from build123d import *

# Parameters (mm, degrees)
SKETCH_1_W          = 30
SKETCH_1_H          = 30
EXTRUDE_1_DEPTH     = 10
SKETCH_4_R          = 1.55
CUT_EXTRUDE_1_DEPTH = 30
SKETCH_5_R          = 3.5
SKETCH_5_R_2        = 1.55
CUT_EXTRUDE_2_DEPTH = 3
SKETCH_6_W          = 30
SKETCH_6_H          = 10
EXTRUDE_2_DEPTH     = 16


with BuildPart() as part:
    # 草图1 → 凸台-拉伸1 (new body)
    with BuildSketch(Plane(origin=(0, 0, 0), x_dir=(1, 0, 0), z_dir=(0, 1, 0))):
        Rectangle(SKETCH_1_W, SKETCH_1_H)
    extrude(amount=EXTRUDE_1_DEPTH)

    # 草图4 → 切除-拉伸1 (cut)
    with BuildSketch(Plane.XZ):
        with Locations(Location((5, 1, 0), (0, 0, 270))):
            Circle(SKETCH_4_R)
        with Locations(Location((5, -9, 0), (0, 0, 270))):
            Circle(SKETCH_4_R)
        with Locations(Location((-5, 1, 0), (0, 0, 270))):
            Circle(SKETCH_4_R)
        with Locations(Location((-5, -9, 0), (0, 0, 270))):
            Circle(SKETCH_4_R)
    extrude(amount=-CUT_EXTRUDE_1_DEPTH, mode=Mode.SUBTRACT)

    # 草图5 → 切除-拉伸2 (cut)
    # profile 1 of 4: a face of its own
    with BuildSketch(Plane.XZ):
        with Locations(Location((5, 1, 0), (0, 0, 270))):
            Circle(SKETCH_5_R)
        with Locations(Location((5, 1, 0), (0, 0, 270))):
            Circle(SKETCH_5_R_2, mode=Mode.SUBTRACT)
    # profile 2 of 4: a face of its own
    with BuildSketch(Plane.XZ):
        with Locations(Location((5, -9, 0), (0, 0, 270))):
            Circle(SKETCH_5_R)
        with Locations(Location((5, -9, 0), (0, 0, 270))):
            Circle(SKETCH_5_R_2, mode=Mode.SUBTRACT)
    # profile 3 of 4: a face of its own
    with BuildSketch(Plane.XZ):
        with Locations(Location((-5, -9, 0), (0, 0, 270))):
            Circle(SKETCH_5_R)
        with Locations(Location((-5, -9, 0), (0, 0, 270))):
            Circle(SKETCH_5_R_2, mode=Mode.SUBTRACT)
    # profile 4 of 4: a face of its own
    with BuildSketch(Plane.XZ):
        with Locations(Location((-5, 1, 0), (0, 0, 270))):
            Circle(SKETCH_5_R)
    extrude(amount=-CUT_EXTRUDE_2_DEPTH, mode=Mode.SUBTRACT)

    # 草图6 → 凸台-拉伸2 (add)
    with BuildSketch(Plane.XY.offset(15)):
        with Locations((0, 5)):
            Rectangle(SKETCH_6_W, SKETCH_6_H)
    extrude(amount=EXTRUDE_2_DEPTH)


solid = part.part
The listing builds one solid part. Answer for the finished solid, in the listing's coordinates (mm). A direction names the side the tool comes from. Coordinates: 2 decimals unless noted, no trailing zeros. Order: outer loops, then holes, each group sorted by start corner. A loop starts at its lowest first (then second) coordinate and runs counter-clockwise, first axis right, second up. Notation, with made-up numbers: (-6.75, 32.5) -> (29.25, 32.5) arc R15 ccw to (29.25, 47.5) -> close; hole circle Ø10 at (77, 50.5). An arc over 180 degrees is marked (long way). Answer in a Markdown table with one row per item. Add a question column.
Item 1: Determine the mould class of faces 1 (the face through (-4.534, 6.451, -0.478)), 2 (the face through (15, 5, 8)), 3 (the face through (-15, 5, 8)), 4 (the face through (0, 10, 8)) for opening direction X: +X half, -X half, draft (parallel to the pull), parting line (faces both ways), or undercut.
Item 2: Which of the six approach directions +Z, -Z, +X, -X, +Y, -Y give full straight-line access (tool end or side, diameter ignored) to faces 5 (the face through (0, 5, 31)), 6 (the face through (-7, 3, -10))?
Item 3: Find section C-C (z = 1). Write down the section's boundary in (x, y).
Item 4: Find section B-B (y = 1.75). Write down the section's boundary in (x, z), then the cut area to 3 significant figures.
Item 5: Find section A-A (x = 5). Write down the section's boundary in (y, z).
Item 6: Find section D-D (y = 4.75). Write down the section's boundary in (x, z).
Item 7: Find the intervals of material crossed by L1, parallel to X at y = 5.75, z = -9; L2, parallel to Z at x = 5.75, y = 7.75; L3, parallel to Z at x = 4.5, y = 1.5, in increasing order. Write a range as from..to.
Item 8: This flat-tipped pin is pushed along its axis until it touches: P1, Ø6.5, axis at x = 5, z = -9, coming from the -Y side. Where does it stop, or does it pass through?
Result set:
| question | item | result |
|---|---|---|
| 1 | face 1 | undercut |
| 1 | face 2 | +X half |
| 1 | face 3 | -X half |
| 1 | face 4 | draft |
| 2 | face 5 | +Z, +X, -X, +Y, -Y |
| 2 | face 6 | -Y |
| 3 | outline | (-15, 0) -> (-8.5, 0) -> (-8.5, 3) -> (-6.55, 3) -> (-6.55, 10) -> (-15, 10) -> close; (-3.45, 3) -> (-1.5, 3) -> (-1.5, 0) -> (1.5, 0) -> (1.5, 3) -> (3.45, 3) -> (3.45, 10) -> (-3.45, 10) -> close; (6.55, 3) -> (8.5, 3) -> (8.5, 0) -> (15, 0) -> (15, 10) -> (6.55, 10) -> close |
| 4 | outline | (-15, -15) -> (15, -15) -> (15, 31) -> (-15, 31) -> close; hole circle Ø7 at (-5, -9); hole circle Ø7 at (-5, 1); hole circle Ø7 at (5, -9); hole circle Ø7 at (5, 1) |
| 4 | area | 1,230 mm² |
| 5 | outline | (0, -15) -> (10, -15) -> (10, -10.55) -> (3, -10.55) -> (3, -12.5) -> (0, -12.5) -> close; (0, -5.5) -> (3, -5.5) -> (3, -7.45) -> (10, -7.45) -> (10, -0.55) -> (3, -0.55) -> (3, -2.5) -> (0, -2.5) -> close; (0, 4.5) -> (3, 4.5) -> (3, 2.55) -> (10, 2.55) -> (10, 31) -> (0, 31) -> close |
| 6 | outline | (-15, -15) -> (15, -15) -> (15, 31) -> (-15, 31) -> close; hole circle Ø3.1 at (-5, -9); hole circle Ø3.1 at (-5, 1); hole circle Ø3.1 at (5, -9); hole circle Ø3.1 at (5, 1) |
| 7 | L1 | x = -15..-6.55, -3.45..3.45, 6.55..15 |
| 7 | L2 | z = -15..-10.36, -7.64..-0.36, 2.36..31 |
| 7 | L3 | z = -15..-12.46, -5.54..-2.46, 4.46..31 |
| 8 | P1 | stops at y = 3 |
